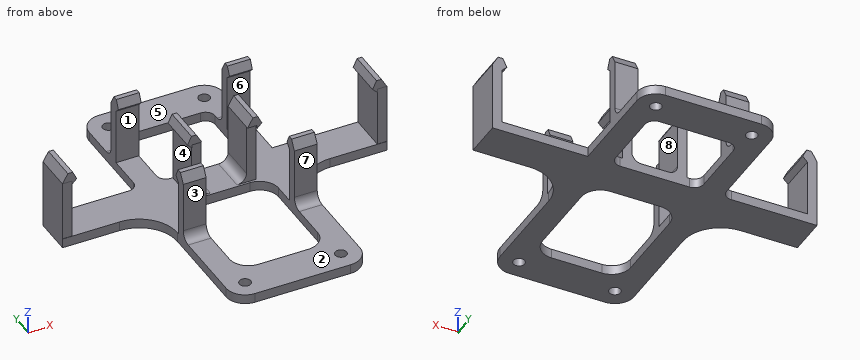
from build123d import *

# Parameters (mm, degrees)
SKETCH1_R           = 1.905
SKETCH1_W           = 29.4132
SKETCH1_H           = 25.4
BOSS_EXTRUDE1_DEPTH = 3.175
SKETCH2_W           = 3.175
SKETCH2_H           = 12.603189316
SKETCH2_H_2         = 11.966378631
SKETCH2_W_2         = 7.62
SKETCH2_H_3         = 3.175
BOSS_EXTRUDE2_DEPTH = 20.1
BOSS_EXTRUDE3_DEPTH = 12.603189
BOSS_EXTRUDE4_DEPTH = 7.62
FILLET1_R           = 6.35
FILLET2_R           = 3.175


with BuildPart() as part:
    # Sketch1 → Boss-Extrude1 (new body)
    with BuildSketch(Plane.XY):
        with BuildLine():
            Line((87.122, 101.406378631), (99.822, 101.406378631))
            Line((99.822, 101.406378631), (119.0752, 101.406378631))
            Line((119.0752, 101.406378631), (131.7752, 101.406378631))
            Line((131.7752, 101.406378631), (131.7752, 63.306378631))
            Line((131.7752, 63.306378631), (163.5252, 63.306378631))
            Line((163.5252, 63.306378631), (163.5252, 50.606378631))
            Line((163.5252, 50.606378631), (144.4752, 50.606378631))
            ThreePointArc((144.4752, 50.606378631), (135.494943879, 46.886634752), (131.7752, 37.906378631))
            Line((131.7752, 37.906378631), (131.7752, 6.35))
            ThreePointArc((131.7752, 6.35), (129.915328061, 1.859871939), (125.4252, 0))
            Line((125.4252, 0), (109.4486, 0))
            Line((109.4486, 0), (93.472, 0))
            ThreePointArc((93.472, 0), (88.981871939, 1.859871939), (87.122, 6.35))
            Line((87.122, 6.35), (87.122, 37.906378631))
            ThreePointArc((87.122, 37.906378631), (83.402256121, 46.886634752), (74.422, 50.606378631))
            Line((74.422, 50.606378631), (55.372, 50.606378631))
            Line((55.372, 50.606378631), (55.372, 63.306378631))
            Line((55.372, 63.306378631), (87.122, 63.306378631))
            Line((87.122, 63.306378631), (87.122, 101.406378631))
        make_face()
        with Locations((93.472, 95.056378631)):
            Circle(SKETCH1_R, mode=Mode.SUBTRACT)
        with Locations((125.4252, 95.056378631)):
            Circle(SKETCH1_R, mode=Mode.SUBTRACT)
        with Locations((93.472, 6.35)):
            Circle(SKETCH1_R, mode=Mode.SUBTRACT)
        with Locations((125.4252, 6.35)):
            Circle(SKETCH1_R, mode=Mode.SUBTRACT)
        with Locations((109.4486, 76.006378631)):
            Rectangle(SKETCH1_W, SKETCH1_H, mode=Mode.SUBTRACT)
        with BuildLine():
            Line((101.092, 50.606378631), (117.8052, 50.606378631))
            ThreePointArc((117.8052, 50.606378631), (122.295328061, 48.746506691), (124.1552, 44.256378631))
            Line((124.1552, 44.256378631), (124.1552, 19.05))
            ThreePointArc((124.1552, 19.05), (122.295328061, 14.559871939), (117.8052, 12.7))
            Line((117.8052, 12.7), (101.092, 12.7))
            ThreePointArc((101.092, 12.7), (96.601871939, 14.559871939), (94.742, 19.05))
            Line((94.742, 19.05), (94.742, 44.256378631))
            ThreePointArc((94.742, 44.256378631), (96.601871939, 48.746506691), (101.092, 50.606378631))
        make_face(mode=Mode.SUBTRACT)
    extrude(amount=BOSS_EXTRUDE1_DEPTH)

    # Sketch2 → Boss-Extrude2 (add)
    with BuildSketch(Plane.XY.offset(3.175)):
        with Locations((56.9595, 57.004783973)):
            Rectangle(SKETCH2_W, SKETCH2_H)
        with Locations((100.2345, 57.323189316)):
            Rectangle(SKETCH2_W, SKETCH2_H_2)
        with Locations((90.932, 35.6775)):
            Rectangle(SKETCH2_W_2, SKETCH2_H_3)
        with Locations((90.932, 79.3525)):
            Rectangle(SKETCH2_W_2, SKETCH2_H_3)
    boss_extrude2 = extrude(amount=BOSS_EXTRUDE2_DEPTH)

    # Sketch3 → Boss-Extrude3 (add)
    with BuildSketch(Plane(origin=(0, 63.306378631, 0), x_dir=(1, 0, 0), z_dir=(0, 1, 0))):
        Polygon((58.547, -22.103427125), (60.1345, -23.690927125), (58.792587105, -26.45), (57.205087105, -26.45), (55.372, -23.275), (58.547, -23.275), align=None)
        Polygon((98.647, -22.103427125), (97.0595, -23.690927125), (98.401412895, -26.45), (99.988912895, -26.45), (101.822, -23.275), (98.647, -23.275), align=None)
    boss_extrude3 = extrude(amount=-BOSS_EXTRUDE3_DEPTH)

    # Sketch4 → Boss-Extrude4 (add)
    with BuildSketch(Plane.ZY.offset(-87.122)):
        Polygon((23.275, 80.94), (23.275, 77.765), (21.982106781, 77.765), (23.569606781, 76.1775), (26.45, 77.519412895), (26.45, 79.106912895), align=None)
        Polygon((26.45, 35.923087105), (23.275, 34.09), (23.275, 37.265), (21.982106781, 37.265), (23.569606781, 38.8525), (26.45, 37.510587105), align=None)
    boss_extrude4 = extrude(amount=-BOSS_EXTRUDE4_DEPTH)

    # Fillet1
    fillet1_edges = [part.edges().sort_by_distance(p)[0] for p in [
        (87.122, 101.406378631, 1.5875),
        (131.7752, 101.406378631, 1.5875),
    ]]
    fillet(fillet1_edges, radius=FILLET1_R)

    # Mirror3: Boss-Extrude2, Boss-Extrude3, Boss-Extrude4 across plane
    add(boss_extrude2.mirror(Plane.ZY.offset(-109.4486)))
    add(boss_extrude3.mirror(Plane.ZY.offset(-109.4486)))
    add(boss_extrude4.mirror(Plane.ZY.offset(-109.4486)))

    # Fillet2
    fillet2_edges = [part.edges().sort_by_distance(p)[0] for p in [
        (101.822, 57.323189315, 3.175),
        (90.932, 34.09, 3.175),
        (90.932, 80.94, 3.175),
        (117.0752, 57.323189315, 3.175),
        (127.9652, 34.09, 3.175),
        (127.9652, 80.94, 3.175),
        (87.122, 63.306378631, 1.5875),
        (94.742, 63.306378631, 1.5875),
        (124.1552, 63.306378631, 1.5875),
        (124.1552, 88.706378631, 1.5875),
        (94.742, 88.706378631, 1.5875),
    ]]
    fillet(fillet2_edges, radius=FILLET2_R)


solid = part.part
Check sheet for the modelled part. Datum: model origin and axes. Units: mm. Face numbers are marked on the shaded views. A direction names the side the tool comes from. Give positions to 0.01 mm unless a question says otherwise; leave off trailing zeros. Loops run counter-clockwise (first coordinate to the right, second up) from the corner with the lowest first, then second, coordinate; pieces in that order, holes last. Notation, with made-up numbers: M -37.5,-21.75 L -27.5,-21.75 A13 ccw -27.5,-6.75 Z; hole C 80,24 d10. An arc over 180 degrees is marked long. Use a Markdown table: item, result. Add a question column.
Q1. Scan lines: line 1 along X through (y, z) = (36.5, 7); line 2 along Y through (x, z) = (94, 9.5) (3 decimals); line 3 along Z through (x, y) = (117, 95) (3 decimals). Record each from-to range of solid material in increasing order. Write a range as [from, to].
Q2. Sectioned sample at C-C, the plane x = 148.5. Record the cut outline in (y, z) (3 decimals).
Q3. Mould release check, pull along Y, two halves, no side actions. Record for the marked faces 1, 2 and 3: pulls with the +Y half, pulls with the -Y half, needs draft (parallel to the pull), parting line crosses it, or undercut.
Q4. Sectioned sample at B-B, the plane y = 70.5. Record the cut outline in (x, z) (3 decimals).
Q5. Go/stop test with flat-tipped pins: pin 1 (1.6 mm diameter, centred on x = 162.5, z = 8.5, fed in from -Y); pin 2 (6 mm diameter, centred on y = 65.5, z = 11.5, fed in from -X); pin 3 (8.5 mm diameter, centred on x = 89.5, z = 14, fed in from -Y); pin 4 (2.5 mm diameter, centred on x = 159, z = 1.5, fed in from -Y). Record where each tip stops, or that it passes through.
Q6. Sectioned sample at D-D, the plane x = 80. Record the cut outline in (y, z) (3 decimals), then the cut area to 3 significant figures.
Q7. Sectioned sample at A-A, the plane z = 20.5. Give the number of separate pieces and of enclosed holes in the cut face, then the cut area to 3 significant figures.
Q8. Tool access check on the marked faces 4, 5, 6, 7 and 8. Record the directions out of +Z, -Z, +X, -X, +Y, -Y that give a thin tool (end or side, any length) a straight path to the whole face; none if there is none.
Verdict:
| question | item | result |
|---|---|---|
| 1 | line 1 | [87.12, 94.74], [124.16, 131.78] |
| 1 | line 2 | [34.09, 37.265], [77.765, 80.94] |
| 1 | line 3 | [0, 3.175] |
| 2 | outline | M 50.606,0 L 63.306,0 L 63.306,3.175 L 50.606,3.175 Z |
| 3 | face 1 | undercut |
| 3 | face 2 | needs draft |
| 3 | face 3 | pulls with the -Y half |
| 4 | outline | M 87.122,0 L 94.742,0 L 94.742,3.175 L 87.122,3.175 Z; M 124.155,0 L 131.775,0 L 131.775,3.175 L 124.155,3.175 Z |
| 5 | pin 1 | y = 50.7 |
| 5 | pin 2 | x = 55.37 |
| 5 | pin 3 | y = 34.09 |
| 5 | pin 4 | y = 50.61 |
| 6 | outline | M 49.316,0 L 63.306,0 L 63.306,3.175 L 49.316,3.175 Z |
| 6 | area | 44.4 mm^2 |
| 7 | separate pieces | 8 |
| 7 | enclosed holes | 0 |
| 7 | area | 253 mm^2 |
| 8 | face 4 | +Y, -Y |
| 8 | face 5 | +Z, +X, -X, +Y |
| 8 | face 6 | +X, -X |
| 8 | face 7 | +Z, +X, -X, -Y |
| 8 | face 8 | +Z, +Y, -Y |
